from build123d import *

# Parameters (mm, degrees)
SKETCH1_W           = 80
SKETCH1_H           = 80
SKETCH1_R           = 3.5
BOSS_EXTRUDE1_DEPTH = 80
SKETCH2_W           = 70
SKETCH2_H           = 75
CUT_EXTRUDE1_DEPTH  = 80
SKETCH3_R           = 2.5
CUT_EXTRUDE2_DEPTH  = 60


with BuildPart() as part:
    # Sketch1 → Boss-Extrude1 (new body)
    with BuildSketch(Plane.XY):
        Rectangle(SKETCH1_W, SKETCH1_H)
        with Locations((0, 15)):
            Circle(SKETCH1_R, mode=Mode.SUBTRACT)
    extrude(amount=BOSS_EXTRUDE1_DEPTH)

    # Sketch2 → Cut-Extrude1 (cut)
    with BuildSketch(Plane(origin=(40, 0, 0), x_dir=(0, 0, -1), z_dir=(1, 0, 0))):
        with Locations((-40, 2.5)):
            Rectangle(SKETCH2_W, SKETCH2_H)
    extrude(amount=-CUT_EXTRUDE1_DEPTH, mode=Mode.SUBTRACT)

    # Sketch3 → Cut-Extrude2 (cut)
    with BuildSketch(Plane.XZ.offset(40)):
        with Locations((-27.5, 67.5)):
            Circle(SKETCH3_R)
        with Locations((7.5, 67.5)):
            Circle(SKETCH3_R)
        with Locations((7.5, 32.5)):
            Circle(SKETCH3_R)
        with Locations((-27.5, 32.5)):
            Circle(SKETCH3_R)
    extrude(amount=-CUT_EXTRUDE2_DEPTH, mode=Mode.SUBTRACT)


solid = part.part
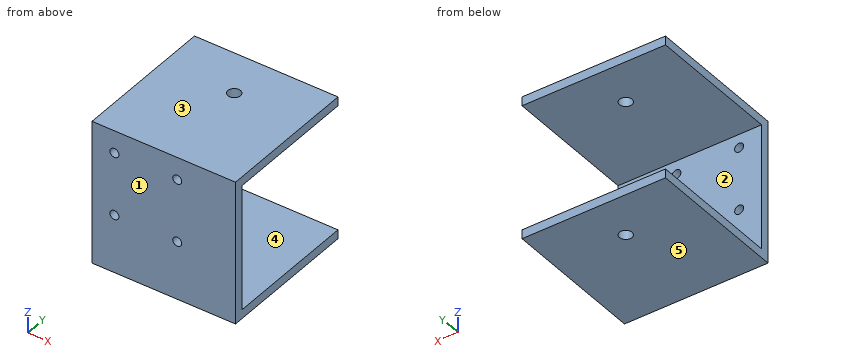
Input: part model. Units: mm. Frame: model coordinates. Face numbers are marked on the shaded views. A direction names the side the tool comes from. Coordinates: 2 decimals unless noted, no trailing zeros. Order: outer loops, then holes, each group sorted by start corner. A loop starts at its lowest first (then second) coordinate and runs counter-clockwise, first axis right, second up. Notation, with made-up numbers: M 5.25,36.5 L 12.25,36.5 A19 ccw 12.25,43.5 Z; hole C 10.25,-3.75 d7. An arc over 180 degrees is marked long. Answer in a Markdown table with one row per item.
(1) Section query C-C, the plane z = 67.5. Output: boundary loops of the cut face in (x, y), plus the area to 3 significant figures.
Numbers:
| item | result |
|---|---|
| outline | M -40,-40 L -30,-40 L -30,-35 L -40,-35 Z; M -25,-40 L 5,-40 L 5,-35 L -25,-35 Z; M 10,-40 L 40,-40 L 40,-35 L 10,-35 Z |
| area | 350 mm^2 |
(2) Access query for the marked faces 1 and 2. Directions: +Z, -Z, +X, -X, +Y, -Y. A direction counts if a zero-diameter tool reaches every point of the face in a straight line with its end or side. Return the directions, or none.
Numbers:
| item | result |
|---|---|
| face 1 | +Z, -Z, +X, -X, -Y |
| face 2 | +X, -X, +Y |
(3) Draft query along Z for the marked faces 3, 4 and 5. Return one class per face: pulls with the +Z half, pulls with the -Z half, needs draft (parallel to the pull), parting line crosses it, or undercut.
Numbers:
| item | result |
|---|---|
| face 3 | pulls with the +Z half |
| face 4 | undercut |
| face 5 | pulls with the -Z half |
(4) Section query B-B, the plane y = -10. Output: boundary loops of the cut face in (x, z).
Numbers:
| item | result |
|---|---|
| outline | M -40,0 L 40,0 L 40,5 L -40,5 Z; M -40,75 L 40,75 L 40,80 L -40,80 Z |
(5) Section query D-D, the plane x = -21.5. Output: boundary loops of the cut face in (y, z).
Numbers:
| item | result |
|---|---|
| outline | M -40,0 L 40,0 L 40,5 L -35,5 L -35,75 L 40,75 L 40,80 L -40,80 Z |
(6) Contact query for flat-ended pins moving along their axis: pin 1 Ø21 at (x, z) = (-17.5, 26.5) entering from +Y; pin 2 Ø6.5 at (x, z) = (-27.5, 67.5) entering from -Y. Output: stop coordinate, or through.
Numbers:
| item | result |
|---|---|
| pin 1 | stops at y = -35 |
| pin 2 | stops at y = -40 |
(7) Material intervals for line 1 (Z direction, x = -27.5, y = -36.8); line 2 (Z direction, x = -23.5, y = -25); line 3 (X direction, y = -36, z = 67), sorted ascending. Write a range as [from, to].
Numbers:
| item | result |
|---|---|
| line 1 | z = [0, 30], [35, 65], [70, 80] |
| line 2 | z = [0, 5], [75, 80] |
| line 3 | x = [-40, -29.95], [-25.05, 5.05], [9.95, 40] |
(8) Section query A-A, the plane x = 7.5. Output: boundary loops of the cut face in (y, z), plus the area to 3 significant figures.
Numbers:
| item | result |
|---|---|
| outline | M -40,0 L 40,0 L 40,5 L -35,5 L -35,30 L -40,30 Z; M -40,35 L -35,35 L -35,65 L -40,65 Z; M -40,70 L -35,70 L -35,75 L 40,75 L 40,80 L -40,80 Z |
| area | 1,100 mm^2 |
